For this review, take the finished solid that the model builds, in its own axes (mm). Face numbers are marked on the shaded views. Round coordinates to 2 decimals unless told otherwise and drop trailing zeros. Loops run counter-clockwise (first coordinate to the right, second up) from the corner with the lowest first, then second, coordinate; pieces in that order, holes last. Notation, with made-up numbers: M -35,83.5 L -27,83.5 A17 ccw -27,89.5 Z; hole C -18,78.5 d8. An arc over 180 degrees is marked long. One line per question, with ' | ' between items. Start each with the question number.
1) Mouldability with a two-part tool opening along Y and no side actions: class the marked faces 1, 2 and 3 as pulls with the +Y half, pulls with the -Y half, needs draft (parallel to the pull), parting line crosses it, or undercut.
2) We need section B-B (x = 0). Give the boundary of the cut face in (y, z).
3) We need section D-D (x = -8). Give the boundary of the cut face in (y, z).
4) For probe 1 along X at (y, z) = (0, -3); probe 2 along Y at (x, z) = (-17, 4.5); probe 3 along X at (y, z) = (3.5, 0.25), list the stretches that pass through material, from the lowest coordinate up. Write a range as from..to.
5) We need section A-A (y = 0). Give the boundary of the cut face in (x, z), and give its area (3 significant figures).
6) We need section C-C (z = 1). Give the boundary of the cut face in (x, y).
7) For pin 1 Ø1.5 at (y, z) = (-17, -2) entering from +X; pin 2 Ø2 at (y, z) = (-8, -1.5) entering from -X; pin 3 Ø1.5 at (x, z) = (13, -1) entering from -Y; pin 4 Ø1.5 at (x, y) = (-13, 11.5) entering from -Z, all flat-tipped, find the tip position at first contact; note any pin that passes through.
Autodesk Inventor part; units mm, degrees
ref_plane "YZ Plane" through (0, 0, 0) normal (1, 0, 0) x (0, 1, 0)
ref_plane "XZ Plane" through (0, 0, 0) normal (0, 1, 0) x (-1, 0, 0)
ref_plane "XY Plane" through (0, 0, 0) normal (0, 0, 1) x (1, 0, 0)
sketch "Sketch1" plane through (0, 0, 0) normal (0, 0, 1) x (1, 0, 0)
  circle A0 centre (0, 0) radius 25 construction
  circle A1 centre (0, 0) radius 21.5
  circle A2 centre (0, 0) radius 19.5
  circle A3 centre (0, 0) radius 19 construction
  circle A4 centre (0, 0) radius 17 construction
  line L0 (25, 0) -> (-25, 0) construction
  line L1 (0, 25) -> (0, -25) construction
  circle A5 centre (-23, 0) radius 2 construction
  circle A6 centre (23, 0) radius 2 construction
  circle A7 centre (0, 19.5) radius 2
  circle A8 centre (0, -19.5) radius 2
  line L2 (-25, 0) -> (-21, 0)
  line L3 (21, 0) -> (25, 0)
  line L4 (0, 21.5) -> (0, 17.5)
  line L5 (0, -17.5) -> (0, -21.5)
  circle A9 centre (22.4059, 0) radius 2
  circle A10 centre (-22.4059, 0) radius 2
  line L6 (-24.4059, 0) -> (-20.4059, 0)
  line L7 (24.4059, 0) -> (20.4059, 0)
  dimension "d6" = 4
  dimension "d0" = 50
  dimension "d2" = 43
  dimension "d3" = 2
  dimension "d4" = 38
  dimension "d5" = 2
  dimension "d7" = 4
  dimension "d8" = 4
  dimension "d9" = 4
  dimension "d22" = 4
extrude "Extrusion1" add sketch "Sketch1" along normal mid plane 10 contours L3 L7 A9 A1 | A1 A9 L7 L3 | A9 A1 A8 A2 A7 | A7 A2 A8 A1 A10 | L4 A2 A7 | A7 A2 L4 | L5 A2 A8 | A8 A2 L5 | A10 L6 L2 A1 | A1 L2 L6 A10 picked at (-0.5203, 20.0925) picked at (0.5115, 20.0968) picked at (0.5115, -20.0968) picked at (-0.5203, -20.0925)
revolve "Revolution1" cut sketch "Sketch1" angle 360 about axis through (-25, 0, 0) along (1, 0, 0) picked at (-22.396, -0.4915) picked at (-21.0251, -0.4685) contours A10 L2 A1 | A1 L2 L6 A10
revolve "Revolution2" cut sketch "Sketch1" angle 360 about axis through (21, 0, 0) along (1, 0, 0) picked at (22.396, -0.4915) picked at (21.0251, -0.4685) contours L3 A9 A1 | A1 A9 L7 L3
revolve "Revolution3" add sketch "Sketch1" angle 360 about axis through (0, 25, 0) along (0, -1, 0) picked at (-0.5203, 20.0925) picked at (-0.3659, 18.8452) contours L4 A2 A7 | A2 L4 A7
revolve "Revolution4" add sketch "Sketch1" angle 360 about axis through (0, 25, 0) along (0, -1, 0) picked at (-0.5203, -20.0925) picked at (-0.3659, -18.8452) contours A8 A2 L5 | A8 L5 A2
properties part number "gimbal_medium_ring"
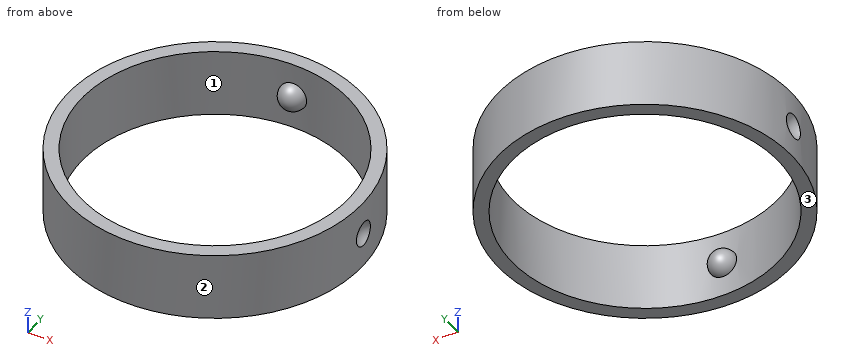
Answers below:
1) face 1: undercut | face 2: parting line crosses it | face 3: needs draft
2) outline: M -21.5,-5 L -19.5,-5 L -19.5,-2 A2 ccw -19.5,2 L -19.5,5 L -21.5,5 Z; M 19.5,-5 L 21.5,-5 L 21.5,5 L 19.5,5 L 19.5,2 A2 ccw 19.5,-2 Z
3) outline: M -19.96,-5 L -17.78,-5 L -17.78,5 L -19.96,5 Z; M 17.78,-5 L 19.96,-5 L 19.96,5 L 17.78,5 Z
4) probe 1: -21.5..-19.5, 19.5..21.5 | probe 2: -13.16..-9.55, 9.55..13.16 | probe 3: -21.21..-19.18, 19.18..21.21
5) outline: M -21.5,-5 L -19.5,-5 L -19.5,5 L -21.5,5 L -21.5,1.78 A2 cw -21.5,-1.78 Z; M 19.5,-5 L 21.5,-5 L 21.5,-1.78 A2 cw 21.5,1.78 L 21.5,5 L 19.5,5 Z | area: 34.4 mm^2
6) outline: M -21.45,-1.45 A21.5 ccw 21.45,-1.45 A1.73 cw 21.45,1.45 A21.5 ccw -21.45,1.45 A1.73 cw Z; hole M -1.73,-19.42 A1.73 cw 1.73,-19.42 A19.5 ccw 1.73,19.42 A1.73 cw -1.73,19.42 A19.5 ccw Z
7) pin 1: x = 14.08 | pin 2: x = -20.33 | pin 3: y = -17.67 | pin 4: through
